from build123d import *

# Parameters (mm, degrees)
BOSS_EXTRUDE1_DEPTH = 100
CUT_EXTRUDE2_DEPTH  = 20
CUT_EXTRUDE3_START  = -20
CUT_EXTRUDE3_DEPTH  = 20
SKETCH9_R           = 40
BOSS_EXTRUDE2_DEPTH = 20
BOSS_EXTRUDE3_START = 20
SKETCH2_R           = 40
BOSS_EXTRUDE3_DEPTH = 20
SKETCH10_R          = 40
BOSS_EXTRUDE6_DEPTH = 20
BOSS_EXTRUDE7_START = 20
SKETCH11_R          = 40
BOSS_EXTRUDE7_DEPTH = 20


with BuildPart() as part:
    # Sketch1 → Boss-Extrude1 (new body)
    with BuildSketch(Plane(origin=(0, 0, 0), x_dir=(0, 0, -1), z_dir=(1, 0, 0))):
        with BuildLine():
            Line((-74.767803634, 0), (-74.767803634, 600))
            ThreePointArc((-74.767803634, 600), (0, 674.767803634), (74.767803634, 600))
            Line((74.767803634, 600), (74.767803634, 0))
            ThreePointArc((74.767803634, 0), (0, -74.767803634), (-74.767803634, 0))
        make_face()
    extrude(amount=BOSS_EXTRUDE1_DEPTH)

    # Sketch8 → Cut-Extrude2 (cut)
    with BuildSketch(Plane.ZY):
        with BuildLine():
            Line((-74.767803634, 600), (-74.767803634, 525))
            Line((-74.767803634, 525), (74.767803634, 525))
            Line((74.767803634, 525), (74.767803634, 600))
            ThreePointArc((74.767803634, 600), (0, 674.767803634), (-74.767803634, 600))
        make_face()
    extrude(amount=-CUT_EXTRUDE2_DEPTH, mode=Mode.SUBTRACT)

    # Sketch7 → Cut-Extrude3 (cut)
    with BuildSketch(Plane(origin=(100, 0, 0), x_dir=(0, 0, -1), z_dir=(1, 0, 0)).offset(CUT_EXTRUDE3_START)):
        with BuildLine():
            Line((-74.767803634, 600), (-74.767803634, 525))
            Line((-74.767803634, 525), (74.767803634, 525))
            Line((74.767803634, 525), (74.767803634, 600))
            ThreePointArc((74.767803634, 600), (0, 674.767803634), (-74.767803634, 600))
        make_face()
    extrude(amount=CUT_EXTRUDE3_DEPTH, mode=Mode.SUBTRACT)

    # Sketch9 → Boss-Extrude2 (add)
    with BuildSketch(Plane.ZY):
        with Locations(Location((0, 0, 0), (0, 0, 180))):
            Circle(SKETCH9_R)
    extrude(amount=BOSS_EXTRUDE2_DEPTH)

    # Sketch2 → Boss-Extrude3 (add)
    with BuildSketch(Plane(origin=(100, 0, 0), x_dir=(0, 0, -1), z_dir=(1, 0, 0)).offset(BOSS_EXTRUDE3_START)):
        Circle(SKETCH2_R)
    extrude(amount=-BOSS_EXTRUDE3_DEPTH)

    # Sketch10 → Boss-Extrude6 (add)
    with BuildSketch(Plane(origin=(80, 0, 0), x_dir=(0, 0, -1), z_dir=(1, 0, 0))):
        with Locations(Location((0, 600, 0), (0, 0, 180))):
            Circle(SKETCH10_R)
    extrude(amount=BOSS_EXTRUDE6_DEPTH)

    # Sketch11 → Boss-Extrude7 (add)
    with BuildSketch(Plane.ZY.offset(-20).offset(BOSS_EXTRUDE7_START)):
        with Locations((0, 600)):
            Circle(SKETCH11_R)
    extrude(amount=-BOSS_EXTRUDE7_DEPTH)


solid = part.part
Source: CAD feature listing. Evaluate the final solid. Frame: model axes, mm. A direction names the side the tool comes from. Give positions to 0.01 mm unless a question says otherwise; leave off trailing zeros. Write each loop counter-clockwise with the first axis right and the second up, starting at its lowest first coordinate (ties: lowest second). Pieces come first, ordered by that corner, then holes. Notation, with made-up numbers: M 89.5,48 L 127.5,48 A18 cw 127.5,52 Z; hole C -10,42.25 d1. An arc over 180 degrees is marked long. Return JSON: item names as keys, results as strings. Group by question number.
1) Pin query (flat end, axial travel): P1, Ø6, axis at x = 85.5, z = -33.5, coming from the +Y side; P2, Ø6, axis at x = 3, y = 575.5, coming from the +Z side; P3, Ø12, axis at y = 168, z = 5, coming from the +X side. Return the tip coordinate at first contact, or that it passes through.
2) Cut plane A-A, the plane x = 7. Output: boundary loops of the cut face in (y, z), plus the area to 3 significant figures.
3) Pull-direction query (Y, two-part tool) for faces 5 (the face through (100, 229, -1)), 6 (the face through (49.3, -74.75, -1.64)), 7 (the face through (20, 568, 32)), 8 (the face through (10, 525, -1)); classes: pulls with the +Y half, pulls with the -Y half, needs draft (parallel to the pull), parting line crosses it, or undercut.
4) Cut plane C-C, the plane y = 193. Output: boundary loops of the cut face in (x, z).
5) Material intervals for line 1 along X through (y, z) = (643, 45); line 2 along X through (y, z) = (162.5, -27.5); line 3 along Z through (x, y) = (72.5, 604.5), sorted ascending. Write a range as [from, to].
6) Cut plane D-D, the plane x = 43. Output: boundary loops of the cut face in (y, z).
7) Set-up query: faces 1 (the face through (80, 568, -32)), 2 (the face through (90, 525, 1)), 3 (the face through (-9.86, -1.76, 39.96)), 4 (the face through (100, 599, -1)). Return all of +Z, -Z, +X, -X, +Y, -Y with unobstructed straight access to the full face (end or side cutting, diameter ignored); none if empty.
8) Cut plane B-B, the plane z = 0. Output: boundary loops of the cut face in (x, y).
Recorded:
{
 "1": {"P1": "stops at y = 625.88", "P2": "stops at z = 33.73", "P3": "stops at x = 100"},
 "2": {"outline": "M 0,-74.77 L 525,-74.77 L 525,74.77 L 0,74.77 A74.77 ccw Z; C 600,0 d80", "area": "92,300 mm²"},
 "3": {"face 5": "needs draft", "face 6": "pulls with the -Y half", "face 7": "undercut", "face 8": "undercut"},
 "4": {"outline": "M 0,-74.77 L 100,-74.77 L 100,74.77 L 0,74.77 Z"},
 "5": {"line 1": "x = [20, 80]", "line 2": "x = [0, 100]", "line 3": "z = [-74.63, 74.63]"},
 "6": {"outline": "M 0,-74.77 L 600,-74.77 A74.77 ccw 600,74.77 L 0,74.77 A74.77 ccw Z"},
 "7": {"face 1": "+X", "face 2": "+Z, -Z, +X", "face 3": "-X", "face 4": "+Z, -Z, +X, +Y"},
 "8": {"outline": "M -20,-40 L 0,-40 L 0,-74.77 L 100,-74.77 L 100,-40 L 120,-40 L 120,40 L 100,40 L 100,525 L 80,525 L 80,560 L 100,560 L 100,640 L 80,640 L 80,674.77 L 20,674.77 L 20,640 L 0,640 L 0,560 L 20,560 L 20,525 L 0,525 L 0,40 L -20,40 Z"}
}
